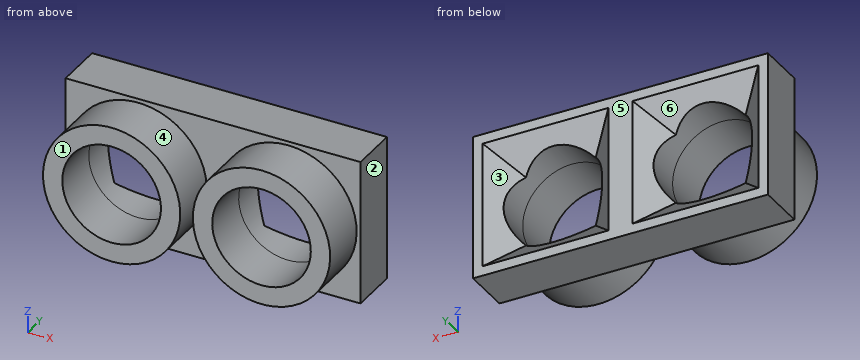
```python
from build123d import *
from build123d.topology import SkipClean

# Parameters (mm, degrees)
SKETCH1_W               = 30.5
SKETCH1_H               = 15
BOSS_EXTRUDE1_DEPTH     = 5
SKETCH2_W               = 13
SKETCH2_H               = 13
CUT_EXTRUDE1_DEPTH      = 3
CHAMFER1_SIZE           = 3
CUT_EXTRUDE3_DEPTH      = 18.257244855
CUT_EXTRUDE3_DEPTH_BACK = 18.257244855
SKETCH4_R               = 5.1
SKETCH5_R               = 7.1
SKETCH5_R_2             = 5.1
BOSS_EXTRUDE3_DEPTH     = 5


with BuildPart() as part:
    # Sketch1 → Boss-Extrude1 (new body)
    with BuildSketch(Plane(origin=(0, 0, 0), x_dir=(1, 0, 0), z_dir=(0, 1, 0))):
        Rectangle(SKETCH1_W, SKETCH1_H)
    extrude(amount=BOSS_EXTRUDE1_DEPTH)

    # Sketch2 → Cut-Extrude1 (cut)
    with BuildSketch(Plane(origin=(0, 5, 0), x_dir=(1, 0, 0), z_dir=(0, 1, 0))):
        with Locations((-7.75, 0)):
            Rectangle(SKETCH2_W, SKETCH2_H)
        with Locations((7.75, 0)):
            Rectangle(SKETCH2_W, SKETCH2_H)
    extrude(amount=-CUT_EXTRUDE1_DEPTH, mode=Mode.SUBTRACT)

    # Chamfer1
    chamfer1_edges = [part.edges().sort_by_distance(p)[0] for p in [
        (-7.75, 2, -6.5),
        (-1.25, 2, 0),
        (-7.75, 2, 6.5),
        (-14.25, 2, 0),
        (7.75, 2, -6.5),
        (14.25, 2, 0),
        (7.75, 2, 6.5),
        (1.25, 2, 0),
    ]]
    chamfer(chamfer1_edges, length=CHAMFER1_SIZE - 0.0001)  # a hair under: the kernel refuses the full size

    # Sketch4 → Cut-Extrude3 (cut, two sides: drawn at the far end of the back side and taken through both)
    with BuildSketch(Plane(origin=(0, 2, 0), x_dir=(1, 0, 0), z_dir=(0, 1, 0)).offset(-CUT_EXTRUDE3_DEPTH_BACK)):
        with Locations(Location((-7.75, 0, 0), (0, 0, 270))):
            Circle(SKETCH4_R)
        with Locations(Location((7.75, 0, 0), (0, 0, 270))):
            Circle(SKETCH4_R)
    extrude(amount=CUT_EXTRUDE3_DEPTH + CUT_EXTRUDE3_DEPTH_BACK, mode=Mode.SUBTRACT)

    # Sketch5 → Boss-Extrude3 (add)
    # profile 1 of 2: a face of its own
    with SkipClean():  # the faces are left unmerged after this step: merging them gives an invalid solid
        with BuildSketch(Plane.XZ):
            with Locations(Location((-7.75, 0, 0), (0, 0, 270))):
                Circle(SKETCH5_R)
            with Locations(Location((-7.75, 0, 0), (0, 0, 45))):
                Circle(SKETCH5_R_2, mode=Mode.SUBTRACT)
        # profile 2 of 2: a face of its own
        with BuildSketch(Plane.XZ):
            with Locations(Location((7.75, 0, 0), (0, 0, 90))):
                Circle(SKETCH5_R)
            with Locations(Location((7.75, 0, 0), (0, 0, 135))):
                Circle(SKETCH5_R_2, mode=Mode.SUBTRACT)
        extrude(amount=BOSS_EXTRUDE3_DEPTH)


solid = part.part
```
Read the model definition and answer for the solid it produces. Units are mm, in the model's axes. Face numbers are marked on the shaded views. A direction names the side the tool comes from. Coordinates: 2 decimals unless noted, no trailing zeros. Write each loop counter-clockwise with the first axis right and the second up, starting at its lowest first coordinate (ties: lowest second). Pieces come first, ordered by that corner, then holes. Notation, with made-up numbers: (82, 6.25) -> (116, 6.25) arc R22 ccw to (116, 24.25) -> close; hole circle Ø11 at (-3.75, 2.25). An arc over 180 degrees is marked (long way). Write item = value, one per line.
(1) Section A-A on y = -2.75 is taken. Write down the section's boundary in (x, z), plus the area to 3 significant figures.
From the geometry:
outline = circle Ø14.2 at (-7.75, 0); circle Ø14.2 at (7.75, 0); hole circle Ø10.2 at (-7.75, 0); hole circle Ø10.2 at (7.75, 0)
area = 153 mm2
(2) Section C-C on z = 0 is taken. Count the separate pieces of the cut face and the enclosed holes in it, plus the area to 3 significant figures.
From the geometry:
separate_pieces = 3
enclosed_holes = 0
area = 86.6 mm2
(3) For a pull along X with two mould halves and no side action, classify the marked faces 1, 2 and 3 as +X half, -X half, draft (parallel to the pull), parting line (faces both ways), or undercut.
From the geometry:
face_1 = draft
face_2 = +X half
face_3 = undercut
(4) Section D-D on y = 3 is taken. Write down the section's boundary in (x, z), plus the area to 3 significant figures.
From the geometry:
outline = (-15.25, -7.5) -> (15.25, -7.5) -> (15.25, 7.5) -> (-15.25, 7.5) -> close; hole (-12.25, -4.5) -> (-10.15, -4.5) arc R5.1 ccw to (-5.35, -4.5) -> (-3.25, -4.5) -> (-3.25, -2.4) arc R5.1 ccw to (-3.25, 2.4) -> (-3.25, 4.5) -> (-5.35, 4.5) arc R5.1 ccw to (-10.15, 4.5) -> (-12.25, 4.5) -> (-12.25, 2.4) arc R5.1 ccw to (-12.25, -2.4) -> close; hole (3.25, -4.5) -> (5.35, -4.5) arc R5.1 ccw to (10.15, -4.5) -> (12.25, -4.5) -> (12.25, -2.4) arc R5.1 ccw to (12.25, 2.4) -> (12.25, 4.5) -> (10.15, 4.5) arc R5.1 ccw to (5.35, 4.5) -> (3.25, 4.5) -> (3.25, 2.4) arc R5.1 ccw to (3.25, -2.4) -> close
area = 280 mm2
(5) Which of the six approach directions +Z, -Z, +X, -X, +Y, -Y give full straight-line access (tool end or side, diameter ignored) to the marked faces 4, 5 and 6?
From the geometry:
face_4 = -Y
face_5 = +Z, -Z, +X, -X, +Y
face_6 = +Y
(6) Given pin 1 Ø4 at (x, z) = (-2.5, -1.5) entering from +Y, flat-ended and moving along its own axis, determine where the tip first touches the part or whether it passes through.
From the geometry:
pin_1 = 5
(7) Straight lines are drawn through the part: L1, parallel to X at y = -3.5, z = 0; L2, parallel to X at y = 0.9, z = 0; L3, parallel to Z at x = -12.5, y = 3.5. For each, find the intervals that lie inside material, in ascending order. Write a range as from..to.
From the geometry:
L1 = -14.85..-12.85, -2.65..-0.65, 0.65..2.65, 12.85..14.85
L2 = -15.25..-12.85, -2.65..2.65, 12.85..15.25
L3 = -7.5..-5, 5..7.5
